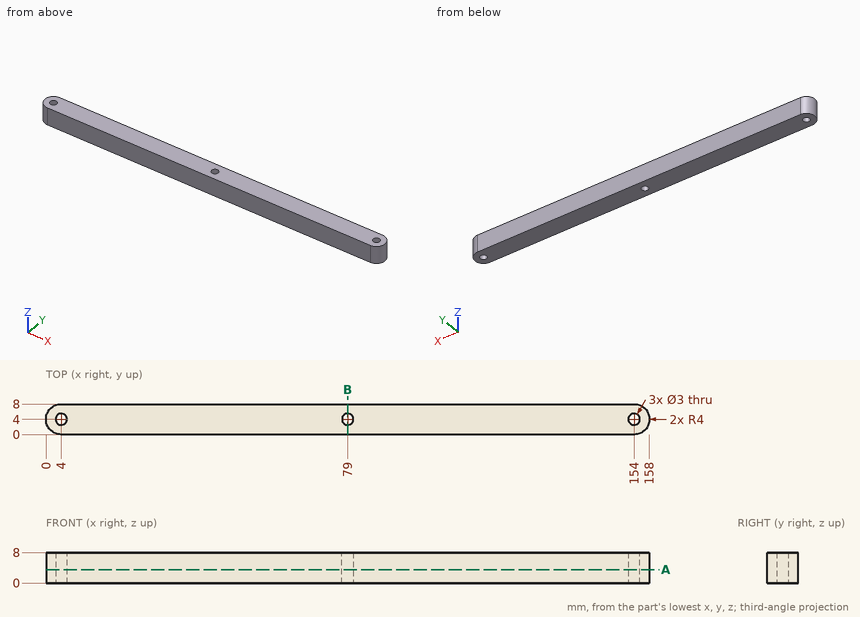
Source: three-view drawing plus pictorial views. Frame: mm from the lowest corner of the part. Give positions to 0.01 mm unless a question says otherwise; leave off trailing zeros. Loops run counter-clockwise (first coordinate to the right, second up) from the corner with the lowest first, then second, coordinate; pieces in that order, holes last.
1) Section query A-A on z = 3.5. Return the cut outline in (x, y), and give its area (3 significant figures).
A:
outline: (4, 0) - (154, 0) arc R4 ccw to (154, 8) - (4, 8) arc R4 ccw to start; hole circle Ø3 at (4, 4); hole circle Ø3 at (79, 4); hole circle Ø3 at (154, 4)
area: 1,230 mm2
2) Line query: L1, parallel to X at y = 4.25, z = 0.5; L2, parallel to Y at x = 79, z = 6.25; L3, parallel to X at y = 3.5, z = 7.25. Output: solid intervals per line, ascending.
A:
L1: x = 0.01 to 2.52, 5.48 to 77.52, 80.48 to 152.52, 155.48 to 157.99
L2: y = 0 to 2.5, 5.5 to 8
L3: x = 0.03 to 2.59, 5.41 to 77.59, 80.41 to 152.59, 155.41 to 157.97
3) Contact query for flat-ended pins moving along their axis: pin 1 (4 mm diameter, centred on x = 4, y = 4, fed in from -Z); pin 2 (2.5 mm diameter, centred on x = 154, y = 4, fed in from -Z). Output: stop coordinate, or through.
A:
pin 1: stops at z = 0
pin 2: passes through
4) Section query B-B on x = 79. Return the cut outline in (y, z), and give its area (3 significant figures).
A:
outline: (0, 0) - (2.5, 0) - (2.5, 8) - (0, 8) - close; (5.5, 0) - (8, 0) - (8, 8) - (5.5, 8) - close
area: 40.0 mm2
